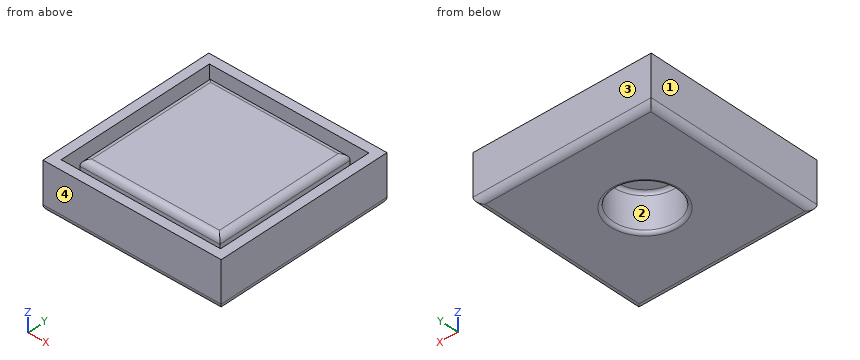
from build123d import *

# Parameters (mm, degrees)
F0_W     = 50.8
F0_H     = 50.8
F0_W_2   = 44.65
F0_H_2   = 44.65
F1_DEPTH = 3
F0_W_3   = 56.8
F0_H_3   = 56.8
F2_DEPTH = 15
F3_R     = 2
F4_R     = 2
F5_R     = 10
F6_DEPTH = 12
F7_R     = 1


with BuildPart() as f1:
    # F0 (on Top) → F1 (new body)
    with BuildSketch(Plane.XY):
        Rectangle(F0_W, F0_H)
        Rectangle(F0_W_2, F0_H_2, mode=Mode.SUBTRACT)
    extrude(amount=F1_DEPTH)

    # F0 (on Top) → F2 (join)
    with BuildSketch(Plane.XY):
        Rectangle(F0_W_3, F0_H_3)
        Rectangle(F0_W, F0_H, mode=Mode.SUBTRACT)
        Rectangle(F0_W_2, F0_H_2)
    extrude(amount=F2_DEPTH)

    # F3
    f3_edges = [f1.edges().sort_by_distance(p)[0] for p in [
        (22.325, 0, 15),
        (0, 22.325, 15),
        (-22.325, 0, 15),
        (0, -22.325, 15),
    ]]
    fillet(f3_edges, radius=F3_R)

    # F4
    f4_edges = [f1.edges().sort_by_distance(p)[0] for p in [
        (28.4, 0, 0),
        (0, 28.4, 0),
        (-28.4, 0, 0),
        (0, -28.4, 0),
    ]]
    fillet(f4_edges, radius=F4_R)

    # F5 (on face) → F6 (cut)
    with BuildSketch(Plane(origin=(0, 0, 0), x_dir=(1, 0, 0), z_dir=(0, 0, -1))):
        Circle(F5_R)
    extrude(amount=-F6_DEPTH, mode=Mode.SUBTRACT)

    # F7
    f7_edges = [f1.edges().sort_by_distance(p)[0] for p in [
        (10, 0, 6),
        (-10, 0, 0),
        (-10, 0, 12),
    ]]
    fillet(f7_edges, radius=F7_R)


solid = f1.part
For this review, take the finished solid that the model builds, in its own axes (mm). Face numbers are marked on the shaded views. Round coordinates to 2 decimals unless told otherwise and drop trailing zeros. Loops run counter-clockwise (first coordinate to the right, second up) from the corner with the lowest first, then second, coordinate; pieces in that order, holes last. Notation, with made-up numbers: (7.5, 62.5) - (23.5, 62.5) arc R18 cw to (23.5, 78.5) - close; hole circle Ø4 at (83, -24). An arc over 180 degrees is marked (long way). Use one line per item in the form item = value.
Item 1: Consider section A-A on z = 9.25. Write out the cut boundary in (x, y) (3 decimals).
Answers:
outline = (-28.4, -28.4) - (28.4, -28.4) - (28.4, 28.4) - (-28.4, 28.4) - close; (-22.325, -22.325) - (22.325, -22.325) - (22.325, 22.325) - (-22.325, 22.325) - close; hole (-25.4, -25.4) - (25.4, -25.4) - (25.4, 25.4) - (-25.4, 25.4) - close; hole circle Ø20 at (0, 0)
Item 2: Clearance check with a flat-ended pin moving along its axis: P1, Ø14.5, axis at x = -1.5, y = -1, coming from the -Z side. State where the tip first meets the part, or that it passes through.
Answers:
P1 = 12
Item 3: Mouldability with a two-part tool opening along Y and no side actions: class the marked faces 1, 2, 3 and 4 as +Y half, -Y half, draft (parallel to the pull), parting line (faces both ways), or undercut.
Answers:
face_1 = draft
face_2 = undercut
face_3 = +Y half
face_4 = -Y half
Item 4: For line 1 (X direction, y = 0, z = 8.5) (3 decimals); line 2 (Y direction, x = -18.5, z = 4.25) (3 decimals), list the stretches that pass through material, from the lowest coordinate up.
Answers:
line_1 = -28.4 to -25.4, -22.325 to -10, 10 to 22.325, 25.4 to 28.4
line_2 = -28.4 to -25.4, -22.325 to 22.325, 25.4 to 28.4
Item 5: Consider section B-B on y = 24. Write out the cut boundary in (x, z).
Answers:
outline = (-28.4, 2) arc R2 ccw to (-26.4, 0) - (26.4, 0) arc R2 ccw to (28.4, 2) - (28.4, 15) - (25.4, 15) - (25.4, 3) - (-25.4, 3) - (-25.4, 15) - (-28.4, 15) - close
Item 6: Consider section C-C on x = 14. Write out the cut boundary in (y, z) (3 decimals), then the cut area to 3 significant figures.
Answers:
outline = (-28.4, 2) arc R2 ccw to (-26.4, 0) - (26.4, 0) arc R2 ccw to (28.4, 2) - (28.4, 15) - (25.4, 15) - (25.4, 3) - (22.325, 3) - (22.325, 13) arc R2 ccw to (20.325, 15) - (-20.325, 15) arc R2 ccw to (-22.325, 13) - (-22.325, 3) - (-25.4, 3) - (-25.4, 15) - (-28.4, 15) - close
area = 775 mm^2
